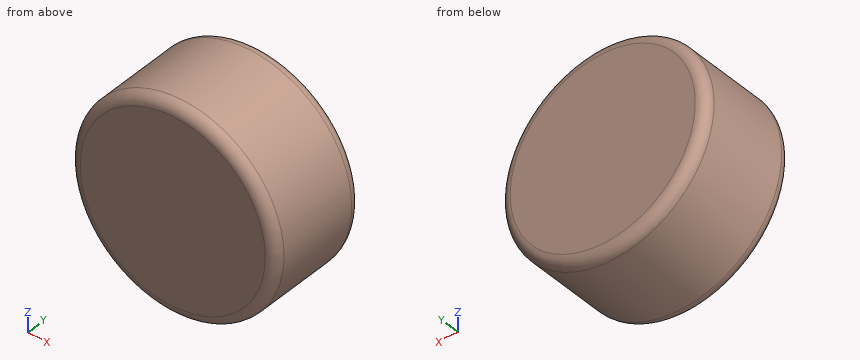
Autodesk Inventor part; units mm, degrees
ref_plane "YZ Plane" through (0, 0, 0) normal (1, 0, 0) x (0, 1, 0)
ref_plane "XZ Plane" through (0, 0, 0) normal (0, 1, 0) x (-1, 0, 0)
ref_plane "XY Plane" through (0, 0, 0) normal (0, 0, 1) x (1, 0, 0)
sketch "Эскиз1" plane through (0, 0, 0) normal (1, 0, 0) x (0, 1, 0)
  line L0 (0, 0) -> (5, 0)
  line L1 (5, 0) -> (5, 5)
  line L2 (5, 5) -> (0, 5)
  line L3 (0, 5) -> (0, 0)
  dimension "d0" = 5
  dimension "d1" = 5
revolve "Вращение1" add sketch "Эскиз1" angle 360 about axis through (0, 0, 0) along (0, 1, 0)
fillet "Сопряжение1" radius 0.5 1 edges at (0, 5, -5)
fillet "Сопряжение2" radius 0.5 1 edges at (0, 0, -5)
properties part number "Магнит2" material "Пластик ПАЭК"
Geometry: final body of the model. Coordinates: model frame, mm. Round coordinates to 2 decimals unless told otherwise and drop trailing zeros. Order: outer loops, then holes, each group sorted by start corner. A loop starts at its lowest first (then second) coordinate and runs counter-clockwise, first axis right, second up. Notation, with made-up numbers: (15, 48) -> (55, 48) arc R22 ccw to (55, 87) -> close; hole circle Ø4 at (77, 38.5). An arc over 180 degrees is marked (long way). Use one line per item in the form item = value. Start each with the question number.
1. Line query: probe 1 along X at (y, z) = (0.4, 2.25); probe 2 along Z at (x, y) = (3, 3); probe 3 along Z at (x, y) = (4.25, 2.9). Output: solid intervals per line, ascending.
2. Cut plane A-A (y = 1.5). Return the cut outline in (x, z).
3. Pin query (flat end, axial travel): pin 1 Ø3 at (x, y) = (-2, 3.5) entering from +Z; pin 2 Ø1.5 at (y, z) = (2, 3.5) entering from +X; pin 3 Ø2 at (x, y) = (-3, 2) entering from +Z. Return the tip coordinate at first contact, or that it passes through.
Solution:
q1.probe_1 = -4.45 to 4.45
q1.probe_2 = -4 to 4
q1.probe_3 = -2.63 to 2.63
q2.outline = circle Ø10 at (0, 0)
q3.pin_1 = 4.97
q3.pin_2 = 4.18
q3.pin_3 = 4.58
